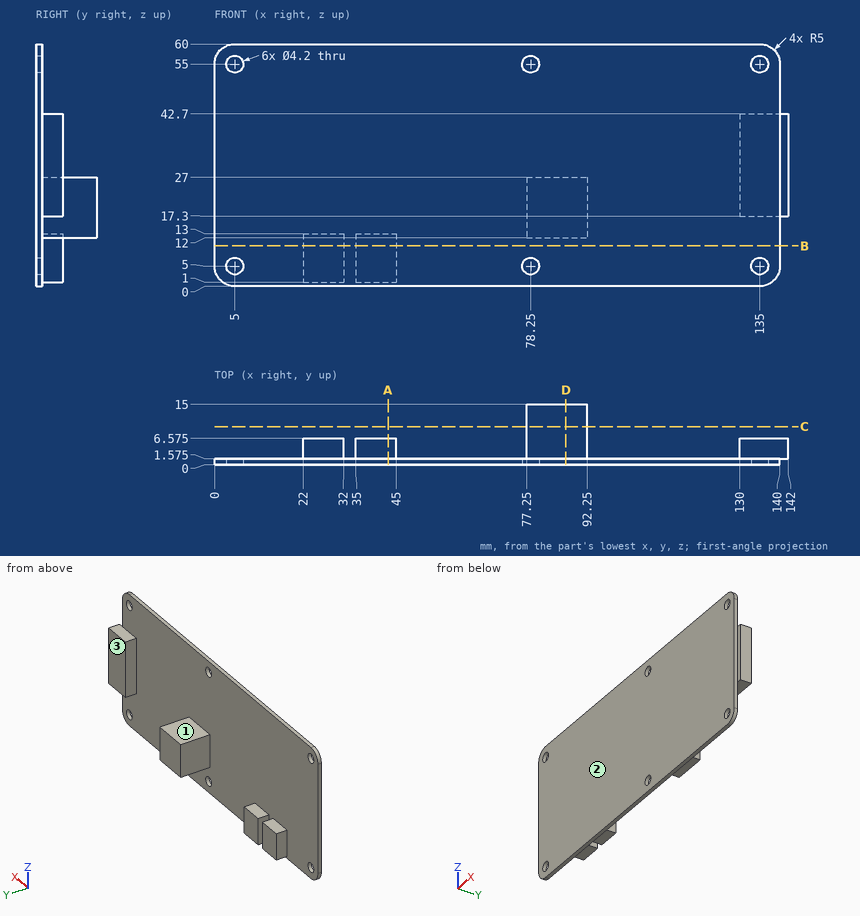
Check sheet for the drawn part. Datum: minimum x, y, z corner. Units: mm. A direction names the side the tool comes from. Give positions to 0.01 mm unless a question says otherwise; leave off trailing zeros. Write each loop counter-clockwise with the first axis right and the second up, starting at its lowest first coordinate (ties: lowest second). Pieces come first, ordered by that corner, then holes.
(1) Gauge pin test, flat ends, axial feed: pin 1 (0.8 mm diameter, centred on y = 1, z = 40.5, fed in from +X); pin 2 (2.5 mm diameter, centred on y = 4.5, z = 9.5, fed in from -X); pin 3 (6 mm diameter, centred on x = 135, z = 24.5, fed in from +Y) (3 decimals); pin 4 (8 mm diameter, centred on y = 9.5, z = 46.5, fed in from +X). Record the tip position at first contact, or that the pin passes through.
(2) Material ranges on line 1 (Z direction, x = 135, y = 0.5); line 2 (X direction, y = 1, z = 55); line 3 (Y direction, x = 108, z = 16) (1 decimal), recorded low to high.
(3) Cross-section at C-C (y = 9.5). Enter the section's corners in (x, z), plus the area to 3 significant figures.
(4) Cross-section at A-A (x = 43). Enter the section's corners in (y, z) (1 decimal).
(5) Cross-section at D-D (x = 87). Enter the section's corners in (y, z) (1 decimal).
(6) Cross-section at B-B (z = 10). Enter the section's corners in (x, y) (1 decimal).
(7) Access from +Z, -Z, +X, -X, +Y, -Y to the whole of each face (thin tool, end or side, straight path). Record for the marked faces 1, 2 and 3.
Worked out:
1. pin 1: stops at x = 140
1. pin 2: stops at x = 22
1. pin 3: stops at y = 6.575
1. pin 4: passes through
2. line 1: z = 0 to 2.9, 7.1 to 52.9, 57.1 to 60
2. line 2: x = 0 to 2.9, 7.1 to 76.15, 80.35 to 132.9, 137.1 to 140
2. line 3: y = 0 to 1.6
3. outline: (77.25, 12) - (92.25, 12) - (92.25, 27) - (77.25, 27) - close
3. area: 225 mm2
4. outline: (0, 0) - (1.6, 0) - (1.6, 1) - (6.6, 1) - (6.6, 13) - (1.6, 13) - (1.6, 60) - (0, 60) - close
5. outline: (0, 0) - (1.6, 0) - (1.6, 12) - (15, 12) - (15, 27) - (1.6, 27) - (1.6, 60) - (0, 60) - close
6. outline: (0, 0) - (140, 0) - (140, 1.6) - (45, 1.6) - (45, 6.6) - (35, 6.6) - (35, 1.6) - (32, 1.6) - (32, 6.6) - (22, 6.6) - (22, 1.6) - (0, 1.6) - close
7. face 1: +Z, -X, +Y
7. face 2: +Z, -Z, +X, -X, -Y
7. face 3: +Z, -Z, +X, +Y
